For this review, use the dimensioned drawing (mm, ordinates from the lowest corner) and the shaded views. A direction names the side the tool comes from. Coordinates: 2 decimals unless noted, no trailing zeros. Write each loop counter-clockwise with the first axis right and the second up, starting at its lowest first coordinate (ties: lowest second). Pieces come first, ordered by that corner, then holes. Notation, with made-up numbers: (39, 69.5) -> (43, 69.5) arc R19 cw to (43, 80.5) -> close; hole circle Ø8 at (83, 70.25). An arc over 180 degrees is marked (long way). Return JSON: item names as keys, results as strings. Group by question number.
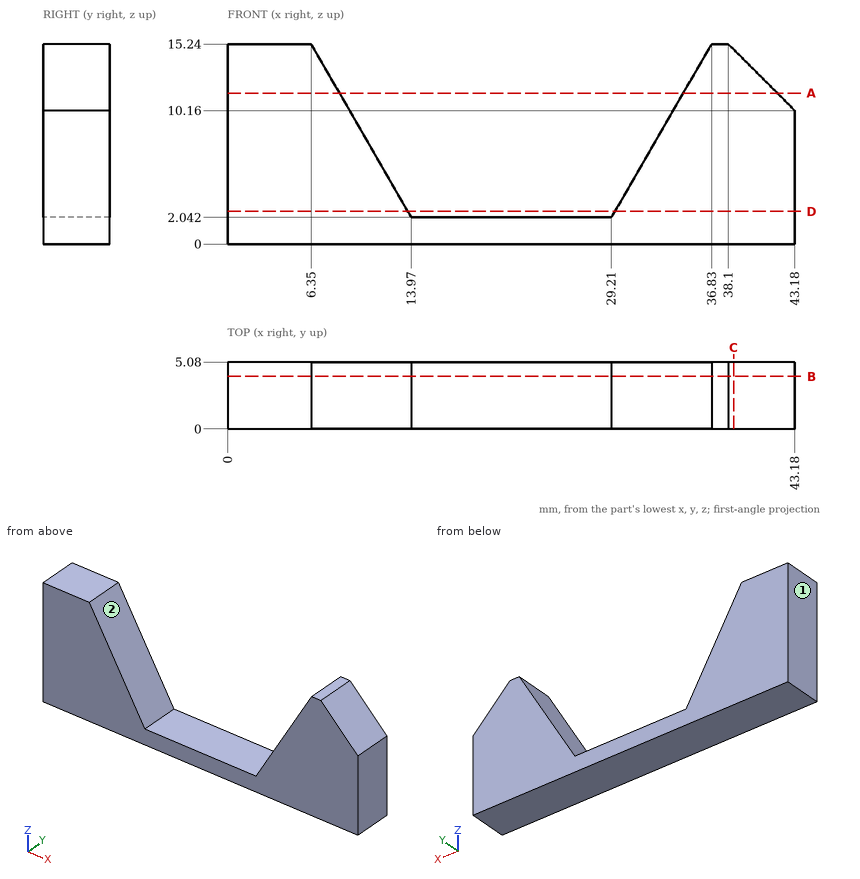
Q1. We need section A-A on z = 11.5. Write out the cut boundary in (x, y).
Q2. For the marked faces 1 and 2, list the 3-axis set-ups (+Z, -Z, +X, -X, +Y, -Y) from which the entire face can be reached by the end or side of a thin tool; tool diameter is ignored.
Q3. For P1, Ø1.5, axis at x = 21, y = 3.5, coming from the -Z side; P2, Ø2, axis at x = 22, y = 3.5, coming from the +Z side, all flat-tipped, find the tip position at first contact; note any pin that passes through.
Q4. We need section C-C on x = 38.5. Write out the cut boundary in (y, z), plus the area to 3 significant figures.
Q5. We need section D-D on z = 2.5. Write out the cut boundary in (x, y) (1 decimal), plus the area to 3 significant figures.
Q6. We need section B-B on y = 4. Write out the cut boundary in (x, z).
Q7. Wall thickness on L1, parallel to Z at x = 26, y = 3.15; L2, parallel to X at y = 1.35, z = 5; L3, parallel to X at y = 3.4, z = 3: over which ranges is each line inside the solid? List them lowest first.
Findings below:
{
 "1": {"outline": "(0, 0) -> (8.51, 0) -> (8.51, 5.08) -> (0, 5.08) -> close; (34.67, 0) -> (41.84, 0) -> (41.84, 5.08) -> (34.67, 5.08) -> close"},
 "2": {"face 1": "+Z, -Z, -X, +Y, -Y", "face 2": "+Z, +Y, -Y"},
 "3": {"P1": "stops at z = 0", "P2": "stops at z = 2.04"},
 "4": {"outline": "(0, 0) -> (5.08, 0) -> (5.08, 14.84) -> (0, 14.84) -> close", "area": "75.4 mm^2"},
 "5": {"outline": "(0, 0) -> (13.7, 0) -> (13.7, 5.1) -> (0, 5.1) -> close; (29.5, 0) -> (43.2, 0) -> (43.2, 5.1) -> (29.5, 5.1) -> close", "area": "139 mm^2"},
 "6": {"outline": "(0, 0) -> (43.18, 0) -> (43.18, 10.16) -> (38.1, 15.24) -> (36.83, 15.24) -> (29.21, 2.04) -> (13.97, 2.04) -> (6.35, 15.24) -> (0, 15.24) -> close"},
 "7": {"L1": "z = 0 to 2.04", "L2": "x = 0 to 12.26, 30.92 to 43.18", "L3": "x = 0 to 13.42, 29.76 to 43.18"}
}
